```python
from build123d import *

# Parameters (mm, degrees)
IZIM1_W               = 346
IZIM1_H               = 501
IZIM1_W_2             = 300
IZIM1_H_2             = 455
TABAN_FLAN_1_DEPTH    = 2
IZIM2_R               = 2.75
KES_EKSTR_ZYON1_DEPTH = 10


# Sheet-metal steps are written as plain solids
with BuildPart() as part:
    # Çizim1 → Taban-Flanş1 (new body)
    with BuildSketch(Plane.XY):
        with Locations((0, -227.5)):
            Rectangle(IZIM1_W, IZIM1_H)
        with Locations((0, -227.5)):
            Rectangle(IZIM1_W_2, IZIM1_H_2, mode=Mode.SUBTRACT)
    extrude(amount=-TABAN_FLAN_1_DEPTH)

    # Çizim2 → Kes-Ekstrüzyon1 (cut)
    with BuildSketch(Plane.XY):
        with Locations((90, 17.5)):
            Circle(IZIM2_R)
        with Locations((-90, 17.5)):
            Circle(IZIM2_R)
        with Locations((-167.5, -62.5)):
            Circle(IZIM2_R)
        with Locations((-167.5, -392.5)):
            Circle(IZIM2_R)
        with Locations(Location((167.5, -392.5, 0), (0, 0, 180))):
            Circle(IZIM2_R)
        with Locations(Location((167.5, -62.5, 0), (0, 0, 180))):
            Circle(IZIM2_R)
        with Locations(Location((90, -472.5, 0), (0, 0, 180))):
            Circle(IZIM2_R)
        with Locations(Location((-90, -472.5, 0), (0, 0, 180))):
            Circle(IZIM2_R)
    extrude(amount=-KES_EKSTR_ZYON1_DEPTH, mode=Mode.SUBTRACT)


solid = part.part
```
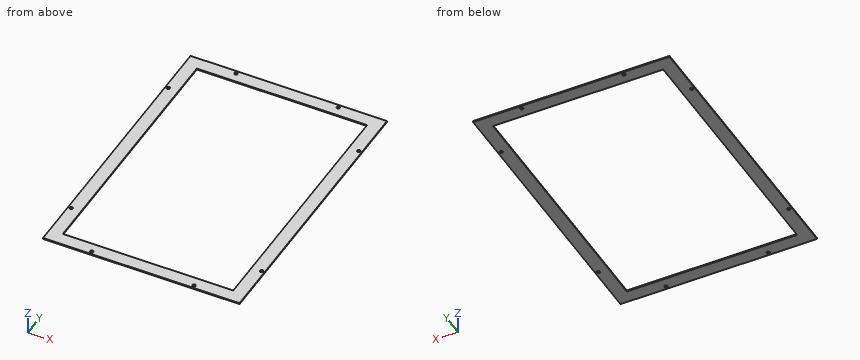
Work out the finished part from the listing and answer in its coordinate system (mm). Coordinates: 2 decimals unless noted, no trailing zeros. Loops run counter-clockwise (first coordinate to the right, second up) from the corner with the lowest first, then second, coordinate; pieces in that order, holes last.
1) Section C-C (x = -116.5) is taken. Give the vertices of the cut face in (y, z).
Results:
outline: (-478, -2) - (-455, -2) - (-455, 0) - (-478, 0) - close; (0, -2) - (23, -2) - (23, 0) - (0, 0) - close
2) Section B-B (z = -0.3) is taken. Give the number of separate pieces and of enclosed holes in the cut face, plus the area to 3 significant figures.
Results:
separate pieces: 1
enclosed holes: 9
area: 36,700 mm2
3) Consider probe 1 along Y at (x, z) = (-167.5, -0.6); probe 2 along Y at (x, z) = (90, -0.85); probe 3 along X at (y, z) = (-392.5, -1). Determine where each line is inside the solid, lowest interval first.
Results:
probe 1: y = -478 to -395.25, -389.75 to -65.25, -59.75 to 23
probe 2: y = -478 to -475.25, -469.75 to -455, 0 to 14.75, 20.25 to 23
probe 3: x = -173 to -170.25, -164.75 to -150, 150 to 164.75, 170.25 to 173
4) A flat-ended cylindrical pin translates along its axis: pin 1 (3.5 mm diameter, centred on x = 90, y = 17.5, fed in from -Z). Find the tip coordinate at first contact, or state that the pin passes through.
Results:
pin 1: passes through
5) Section A-A (y = -229) is taken. Give the vertices of the cut face in (x, z), plus the area to 3 significant figures.
Results:
outline: (-173, -2) - (-150, -2) - (-150, 0) - (-173, 0) - close; (150, -2) - (173, -2) - (173, 0) - (150, 0) - close
area: 92.0 mm2
